Autodesk Inventor part; units mm, degrees
ref_plane "YZ Plane" through (0, 0, 0) normal (1, 0, 0) x (0, 1, 0)
ref_plane "XZ Plane" through (0, 0, 0) normal (0, 1, 0) x (-1, 0, 0)
ref_plane "XY Plane" through (0, 0, 0) normal (0, 0, 1) x (1, 0, 0)
sketch "Sketch1" plane through (0, 0, 0) normal (0, 0, 1) x (1, 0, 0)
  circle A0 centre (0, 0) radius 27
  dimension "d0" = 54
extrude "Extrusion1" add sketch "Sketch1" along normal blind 246
sketch "Sketch2" plane through (0, 0, 246) normal (0, 0, 1) x (1, 0, 0)
  circle A0 centre (0, 0) radius 25.3
  dimension "d3" = 50.6
extrude "Extrusion2" cut sketch "Sketch2" against normal through all
sketch "Sketch3" plane through (0, 0, 0) normal (0, 1, 0) x (-1, 0, 0)
  line L0 (0, 0) -> (0, 246)
  line L1 (0, 246) -> (0, 186)
  line L2 (0, 0) -> (0, 70)
  circle A0 centre (0, 186) radius 1.5
  circle A1 centre (0, 70) radius 1.5
  dimension "d6" = 60
  dimension "d7" = 246
  dimension "d8" = 70
  dimension "d9" = 3
extrude "Extrusion3" cut sketch "Sketch3" against normal through all
pattern_circular "Circular Pattern2" count 2 over 144 about axis through (0, 0, -10) along (0, 0, -1) of "Extrusion3"
properties part number "2207_Cu Tube_V1"
Build history of the part. All positions in model axes, mm. Round coordinates to 2 decimals unless told otherwise and drop trailing zeros. Write each loop counter-clockwise with the first axis right and the second up, starting at its lowest first coordinate (ties: lowest second). Pieces come first, ordered by that corner, then holes. Notation, with made-up numbers: M 86,1.25 L 96,1.25 A19 cw 96,35.25 Z; hole C 57,69.5 d8. An arc over 180 degrees is marked long. Use CSV: the item, a comma, the result in double quotes.
1. Saw through at A-A (y = 0). Give the cut face in (x, z), plus the area to 3 significant figures.
Reply:
outline,"M -27,0 L -25.3,0 L -25.3,246 L -27,246 Z; M 25.3,0 L 27,0 L 27,246 L 25.3,246 Z"
area,"836 mm²"
2. Two-plate mould, pull along Y, no slides. Class faces 1 (the face through (-5.48, -24.7, 124.72)), 2 (the face through (-5.85, 26.36, 121.28)), 3 (the face through (-8.13, 24.13, 246)): +Y half, -Y half, draft (parallel to the pull), parting line (faces both ways), or undercut.
Reply:
face 1,"undercut"
face 2,"parting line"
face 3,"draft"
3. Flat gauge pins, fed straight in: pin 1 (5 mm diameter, centred on x = -18, z = 160.5, fed in from +Y); pin 2 (2.5 mm diameter, centred on x = 0, z = 186, fed in from -Y); pin 3 (4 mm diameter, centred on x = 0, z = 70, fed in from +Y). Where does each tip first touch, or does it go through?
Reply:
pin 1,"stops at y = 22.11"
pin 2,"stops at y = 25.27"
pin 3,"stops at y = 27"
4. Saw through at B-B (x = -10.5). Give the cut face in (y, z), plus the area to 3 significant figures.
Reply:
outline,"M -24.87,0 L -23.02,0 L -23.02,246 L -24.87,246 Z; M 23.02,0 L 24.87,0 L 24.87,246 L 23.02,246 Z"
area,"913 mm²"
5. Saw through at C-C (z = 230). Give the cut face in (x, y), plus the area to 3 significant figures.
Reply:
outline,"C 0,0 d54; hole C 0,0 d50.6"
area,"279 mm²"
6. Wall check: probe 1 along Z at (x, y) = (0, -26.5); probe 2 along Y at (x, z) = (0, 166.5); probe 3 along X at (y, z) = (16, 154). Give the ranges that are in metal, low to high. Write a range as from..to.
Reply:
probe 1,"z = 0..68.5, 71.5..184.5, 187.5..246"
probe 2,"y = -27..-25.3, 25.3..27"
probe 3,"x = -21.75..-19.6, 19.6..21.75"
